CAD build for the part. Positions are in the model's coordinates, mm. A direction names the side the tool comes from. Give positions to 0.01 mm unless a question says otherwise; leave off trailing zeros. Order: outer loops, then holes, each group sorted by start corner. A loop starts at its lowest first (then second) coordinate and runs counter-clockwise, first axis right, second up. Notation, with made-up numbers: M 54,16 L 66,16 A20 ccw 66,39 Z; hole C 26.5,35 d6. An arc over 180 degrees is marked long. Put each result on its own line as item: value. Start each with the question number.
1) Cut at B-B (z = -24.1). Write the cut outline in (x, y).
2) Two-plate mould, pull along Z, no slides. Class faces 1 (the face through (65.897, -4.582, 28.528)), 2 (the face through (-1, 2, -30.5)), 3 (the face through (-7.1, 18.8, 22.2)): released by +Z, released by -Z, zero draft, split by the parting line, or undercut.
3) Cut at C-C (x = 0). Write the cut outline in (y, z), and give its area (3 significant figures).
4) Pin check, flat tips, straight feed: pin 1 (1.6 mm diameter, centred on y = 31.5, z = 18.5, fed in from +X); pin 2 (2 mm diameter, centred on x = -34, z = 21, fed in from +Y); pin 3 (5 mm diameter, centred on x = -20.48, y = 34.85, fed in from +Z). Stop position of each tip, or through.
5) Cut at A-A (y = 4.65). Write the cut outline in (x, z).
6) Cut at D-D (z = -4). Write the cut outline in (x, y).
7) Drill centre lines: line 1 (Z direction, x = -6, y = 19); line 2 (X direction, y = 19, z = 21); line 3 (Y direction, x = 69.5, z = -23). Where is each one in solid material? Low to high. Write a range as [from, to].
8) Tool access for faces 4 (the face through (-69, 30, 17)), 5 (the face through (1, 17.25, 0)), 6 (the face through (-43.5, -11, -28)), 7 (the face through (58.65, 18.77, 23.24)), 8 (the face through (-55.42, -18.77, 21.18)): list every direction of +Z, -Z, +X, -X, +Y, -Y with a clear straight run to the whole face (end or side of a thin tool).
```python
from build123d import *

# Parameters (mm, degrees)
SKETCH1_W           = 151
SKETCH1_H           = 61
SKETCH1_W_2         = 143
SKETCH1_H_2         = 53
BOSS_EXTRUDE1_DEPTH = 20.25
SKETCH2_W           = 143
SKETCH2_H           = 53
BOSS_EXTRUDE2_DEPTH = 3
SKETCH7_W           = 53
SKETCH7_H           = 37.5
CUT_EXTRUDE3_DEPTH  = 4
SKETCH9_W           = 147
SKETCH9_H           = 53
BOSS_EXTRUDE3_DEPTH = 3
CUT_EXTRUDE4_REACH  = 92.944
SKETCH10_R          = 1.6
SKETCH12_R          = 1.55
CUT_EXTRUDE6_DEPTH  = 100.152975245
SKETCH13_W          = 7
SKETCH13_H          = 19.36
BOSS_EXTRUDE4_DEPTH = 2
SKETCH16_R          = 1.6
CUT_EXTRUDE7_DEPTH  = 10
SKETCH17_W          = 7
SKETCH17_H          = 15
SKETCH17_R          = 2
BOSS_EXTRUDE5_DEPTH = 3
SKETCH18_R          = 1.6
CUT_EXTRUDE8_DEPTH  = 10
SKETCH19_W          = 25
SKETCH19_H          = 12
CUT_EXTRUDE9_DEPTH  = 105.834164756


with BuildPart() as part:
    # Sketch1 → Boss-Extrude1 (new, symmetric)
    with BuildSketch(Plane(origin=(0, 0, 0), x_dir=(1, 0, 0), z_dir=(0, 1, 0))):
        Rectangle(SKETCH1_W, SKETCH1_H)
        Rectangle(SKETCH1_W_2, SKETCH1_H_2, mode=Mode.SUBTRACT)
    extrude(amount=BOSS_EXTRUDE1_DEPTH, both=True)

    # Sketch2 → Boss-Extrude2 (add)
    with BuildSketch(Plane.XZ.offset(20.25)):
        Rectangle(SKETCH2_W, SKETCH2_H)
    extrude(amount=-BOSS_EXTRUDE2_DEPTH)

    # Sketch7 → Cut-Extrude3 (cut)
    with BuildSketch(Plane(origin=(75.5, 0, 0), x_dir=(0, 0, -1), z_dir=(1, 0, 0))):
        with Locations((0, 1.5)):
            Rectangle(SKETCH7_W, SKETCH7_H)
    extrude(amount=-CUT_EXTRUDE3_DEPTH, mode=Mode.SUBTRACT)

    # Sketch9 → Boss-Extrude3 (add)
    with BuildSketch(Plane(origin=(0, 20.25, 0), x_dir=(1, 0, 0), z_dir=(0, 1, 0))):
        with Locations((2, 0)):
            Rectangle(SKETCH9_W, SKETCH9_H)
    extrude(amount=-BOSS_EXTRUDE3_DEPTH)

    # Sketch10 → Cut-Extrude4 (cut, up to next)
    with BuildSketch(Plane(origin=(0, 20.25, 0), x_dir=(1, 0, 0), z_dir=(0, 1, 0)), mode=Mode.PRIVATE) as cut_extrude4_sk1:
        with Locations(Location((60, 24.1, 0), (0, 0, 270))):
            Circle(SKETCH10_R)
    cut_extrude4_tool1 = extrude(cut_extrude4_sk1.sketch, amount=-CUT_EXTRUDE4_REACH, mode=Mode.PRIVATE) & part.part
    # Sketch10 → Cut-Extrude4 (cut, up to next)
    with BuildSketch(Plane(origin=(0, 20.25, 0), x_dir=(1, 0, 0), z_dir=(0, 1, 0)), mode=Mode.PRIVATE) as cut_extrude4_sk2:
        with Locations(Location((60, -24.1, 0), (0, 0, 90))):
            Circle(SKETCH10_R)
    cut_extrude4_tool2 = extrude(cut_extrude4_sk2.sketch, amount=-CUT_EXTRUDE4_REACH, mode=Mode.PRIVATE) & part.part
    # Sketch10 → Cut-Extrude4 (cut, up to next)
    with BuildSketch(Plane(origin=(0, 20.25, 0), x_dir=(1, 0, 0), z_dir=(0, 1, 0)), mode=Mode.PRIVATE) as cut_extrude4_sk3:
        with Locations(Location((-6.04, 21, 0), (0, 0, 270))):
            Circle(SKETCH10_R)
    cut_extrude4_tool3 = extrude(cut_extrude4_sk3.sketch, amount=-CUT_EXTRUDE4_REACH, mode=Mode.PRIVATE) & part.part
    # Sketch10 → Cut-Extrude4 (cut, up to next)
    with BuildSketch(Plane(origin=(0, 20.25, 0), x_dir=(1, 0, 0), z_dir=(0, 1, 0)), mode=Mode.PRIVATE) as cut_extrude4_sk4:
        with Locations(Location((-6.04, -21, 0), (0, 0, 90))):
            Circle(SKETCH10_R)
    cut_extrude4_tool4 = extrude(cut_extrude4_sk4.sketch, amount=-CUT_EXTRUDE4_REACH, mode=Mode.PRIVATE) & part.part
    add(cut_extrude4_tool1.solids().sort_by_distance((60, 20.25, -24.1))[0], mode=Mode.SUBTRACT)
    add(cut_extrude4_tool2.solids().sort_by_distance((60, 20.25, 24.1))[0], mode=Mode.SUBTRACT)
    add(cut_extrude4_tool3.solids().sort_by_distance((-6.04, 20.25, -21))[0], mode=Mode.SUBTRACT)
    add(cut_extrude4_tool4.solids().sort_by_distance((-6.04, 20.25, 21))[0], mode=Mode.SUBTRACT)

    # Sketch12 → Cut-Extrude6 (cut, through all)
    with BuildSketch(Plane.XY.offset(30.5)):
        with Locations((67.445205237, 4.65)):
            Circle(SKETCH12_R)
        with Locations((67.445205237, -4.65)):
            Circle(SKETCH12_R)
        with Locations((17.545205237, 4.65)):
            Circle(SKETCH12_R)
        with Locations((17.545205237, -4.65)):
            Circle(SKETCH12_R)
    extrude(amount=-CUT_EXTRUDE6_DEPTH, mode=Mode.SUBTRACT)

    # Sketch13 → Boss-Extrude4 (add)
    with BuildSketch(Plane.XY.offset(17)):
        with Locations((-69.37, 29.93)):
            Rectangle(SKETCH13_W, SKETCH13_H)
    boss_extrude4 = extrude(amount=BOSS_EXTRUDE4_DEPTH)

    # Sketch16 → Cut-Extrude7 (cut)
    with BuildSketch(Plane.XY.offset(19)):
        with Locations((-69.262241782, 24.85)):
            Circle(SKETCH16_R)
        with Locations((-69.262241782, 34.85)):
            Circle(SKETCH16_R)
    cut_extrude7 = extrude(amount=-CUT_EXTRUDE7_DEPTH, mode=Mode.SUBTRACT)

    # Mirror1: Boss-Extrude4, Cut-Extrude7 across plane
    add(boss_extrude4.mirror(Plane(origin=(-44.87, 0, 0), x_dir=(0, 0, 1), z_dir=(1, 0, 0))))
    add(cut_extrude7.mirror(Plane(origin=(-44.87, 0, 0), x_dir=(0, 0, 1), z_dir=(1, 0, 0))), mode=Mode.SUBTRACT)

    # Sketch17 → Boss-Extrude5 (add)
    with BuildSketch(Plane(origin=(0, 0, -30.5), x_dir=(-1, 0, 0), z_dir=(0, 0, -1))):
        with Locations((55.31, 27.75)):
            Rectangle(SKETCH17_W, SKETCH17_H)
        with Locations((55.31, 30.15)):
            Circle(SKETCH17_R, mode=Mode.SUBTRACT)
    extrude(amount=-BOSS_EXTRUDE5_DEPTH)

    # Sketch18 → Cut-Extrude8 (cut)
    with BuildSketch(Plane.XZ.offset(20.25)):
        with Locations(Location((-56.5, 20, 0), (0, 0, 270))):
            Circle(SKETCH18_R)
        with Locations(Location((-56.5, -20, 0), (0, 0, 270))):
            Circle(SKETCH18_R)
    extrude(amount=-CUT_EXTRUDE8_DEPTH, mode=Mode.SUBTRACT)

    # Sketch19 → Cut-Extrude9 (cut, through all)
    with BuildSketch(Plane.XY.offset(30.5)):
        with Locations((-56, -11.25)):
            Rectangle(SKETCH19_W, SKETCH19_H)
    extrude(amount=-CUT_EXTRUDE9_DEPTH, mode=Mode.SUBTRACT)


solid = part.part
```
Solution:
1. outline: M -75.5,-20.25 L 75.5,-20.25 L 75.5,-17.25 L -71.5,-17.25 L -71.5,17.25 L 58.4,17.25 L 58.4,20.25 L -75.5,20.25 Z; M 61.6,17.25 L 75.5,17.25 L 75.5,20.25 L 61.6,20.25 Z
2. face 1: zero draft
2. face 2: released by -Z
2. face 3: undercut
3. outline: M -20.25,-30.5 L 20.25,-30.5 L 20.25,30.5 L -20.25,30.5 Z; hole M -17.25,-26.5 L 17.25,-26.5 L 17.25,26.5 L -17.25,26.5 Z
3. area: 642 mm²
4. pin 1: x = -16.87
4. pin 2: y = 20.25
4. pin 3: z = 19
5. outline: M -75.5,-30.5 L 16,-30.5 L 16,-26.5 L -71.5,-26.5 L -71.5,26.5 L 16,26.5 L 16,30.5 L -75.5,30.5 Z; M 19.1,-30.5 L 65.9,-30.5 L 65.9,-26.5 L 19.1,-26.5 Z; M 19.1,26.5 L 65.9,26.5 L 65.9,30.5 L 19.1,30.5 Z; M 69,-30.5 L 75.5,-30.5 L 75.5,-26.5 L 69,-26.5 Z; M 69,26.5 L 75.5,26.5 L 75.5,30.5 L 69,30.5 Z
6. outline: M -75.5,-20.25 L 75.5,-20.25 L 75.5,-17.25 L -71.5,-17.25 L -71.5,17.25 L 75.5,17.25 L 75.5,20.25 L -75.5,20.25 Z
7. line 1: [-30.5, -22.6], [-19.4, 19.4], [22.6, 30.5]
7. line 2: [-75.5, -7.64], [-4.44, 75.5]
7. line 3: [-20.25, -17.25], [17.25, 20.25]
8. face 4: -Z, +X, -X, +Y
8. face 5: +X
8. face 6: +Z, -Z
8. face 7: +Y
8. face 8: -Y
